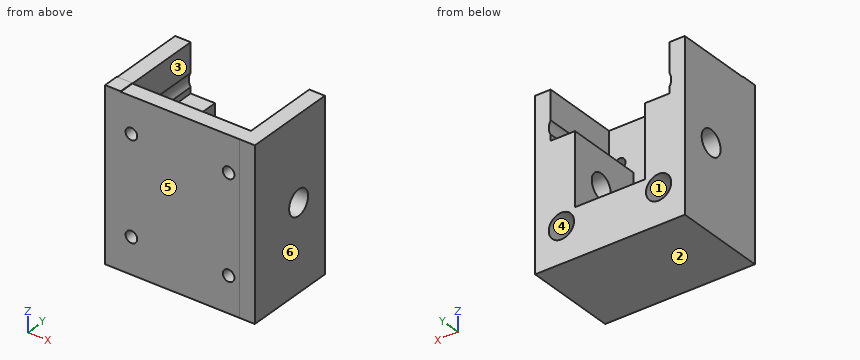
Autodesk Inventor part; units mm, degrees
ref_plane "Work Plane1" through (-15.25, 11.25, -51.1) normal (0, 1, 0) x (1, 0, 0)
ref_plane "Work Plane2" through (-15.25, 11.25, -7.7) normal (-1, 0, 0) x (0, 0, 1)
ref_plane "Work Plane3" through (15.25, 11.25, -51.1) normal (1, 0, 0) x (0, 0, -1)
ref_plane "Work Plane1" through (-15.25, 11.25, -51.1) normal (0, 1, 0) x (1, 0, 0)
sketch "Sketch1" plane through (-15.25, 11.25, -51.1) normal (0, 1, 0) x (1, 0, 0)
  line L0 (0, 0) -> (-1, 0)
  line L1 (30.5, 0) -> (30.5, -43.4)
  line L2 (0, 0) -> (30.5, 0)
  line L3 (30.5, 0) -> (30.5, -43.4)
  line L4 (30.5, -43.4) -> (0, -43.4)
  line L5 (0, -43.4) -> (0, 0)
  circle A0 centre (2.75, -9.2) radius 1.5
  circle A1 centre (2.75, -9.2) radius 1.5
  circle A2 centre (2.75, -34.2) radius 1.5
  circle A3 centre (2.75, -34.2) radius 1.5
  circle A4 centre (27.75, -34.2) radius 1.5
  circle A5 centre (27.75, -34.2) radius 1.5
  circle A6 centre (27.75, -9.2) radius 1.5
  circle A7 centre (27.75, -9.2) radius 1.5
  point P0 (15.25, -51.1)
extrude "Extrusion1" add sketch "Sketch1" along normal blind 4
ref_plane "Work Plane2" through (-15.25, 11.25, -7.7) normal (-1, 0, 0) x (0, 0, 1)
sketch "Sketch2" plane through (-15.25, 11.25, -7.7) normal (-1, 0, 0) x (0, 0, 1)
  line L0 (-43.4, 0) -> (-43.4, 4)
  line L1 (-43.4, 0) -> (0.1445, 0)
  line L2 (0.1445, 0) -> (0.1445, 4)
  line L3 (0.1445, 4) -> (-43.4, 4)
  line L4 (-43.4, 4) -> (-43.4, 0)
  point P0 (7.7, -11.25)
extrude "Extrusion2" add sketch "Sketch2" along normal blind 4
ref_plane "Work Plane3" through (15.25, 11.25, -51.1) normal (1, 0, 0) x (0, 0, -1)
sketch "Sketch3" plane through (15.25, 11.25, -51.1) normal (1, 0, 0) x (0, 0, -1)
  line L0 (0, 0) -> (0, 4)
  line L1 (0, 4) -> (-43.4, 4)
  line L2 (-43.4, 4) -> (-43.4, 0.0024)
  line L3 (-43.4, 0.0024) -> (0, 0.0024)
  line L4 (0, 0.0024) -> (0, 4)
  point P0 (-51.1, -11.25)
extrude "Extrusion3" add sketch "Sketch3" along normal blind 4
ref_plane "Work Plane6" through (-15.25, 15.25, -51.1) normal (0, 1, 0) x (1, 0, 0)
sketch "Sketch4" plane through (-15.25, 15.25, -51.1) normal (0, 1, 0) x (1, 0, 0)
  line L0 (-0.75, -43.4) -> (0.25, -43.4)
  line L1 (-0.0048, -43.4) -> (-4, -43.4)
  line L2 (-4, -43.4) -> (-4, 0)
  line L3 (-4, 0) -> (-0.0048, 0)
  line L4 (-0.0048, 0) -> (-0.0048, -43.4)
  point P0 (15.25, -51.1)
extrude "Extrusion4" add sketch "Sketch4" along normal blind 15
ref_plane "Work Plane5" through (-15.25, 15.25, -51.1) normal (0, 1, 0) x (1, 0, 0)
sketch "Sketch5" plane through (-15.25, 15.25, -51.1) normal (0, 1, 0) x (1, 0, 0)
  line L0 (30.5, 0) -> (34.5, 0)
  line L1 (30.5, -43.4) -> (30.5, 0)
  line L2 (34.5, 0) -> (30.5, 0)
  line L3 (30.5, 0) -> (30.5, -43.4)
  line L4 (30.5, -43.4) -> (34.5, -43.4)
  line L5 (34.5, -43.4) -> (34.5, 0)
  point P0 (15.25, -51.1)
extrude "Extrusion5" add sketch "Sketch5" along normal blind 15
ref_plane "Work Plane4" through (-15.25, 15.25, -51.1) normal (0, 1, 0) x (1, 0, 0)
sketch "Sketch6" plane through (-15.25, 15.25, -51.1) normal (0, 1, 0) x (1, 0, 0)
  circle A0 centre (2.75, -34.2) radius 2
  circle A1 centre (2.75, -34.2) radius 3.25
  circle A2 centre (27.75, -34.2) radius 1.5
  circle A3 centre (27.75, -34.2) radius 3.25
  circle A4 centre (27.75, -9.2) radius 1.5
  circle A5 centre (27.75, -9.2) radius 3.25
  circle A6 centre (2.75, -9.2) radius 1.5
  circle A7 centre (2.75, -9.2) radius 3.25
  line L0 (15.25, -21.7) -> (24.25, -21.7)
  line L1 (15.25, -21.7) -> (6.25, -21.7)
  line L2 (30.5, 0) -> (30.5, -43.4)
  line L3 (24.25, -21.7) -> (30.5, -21.7)
  line L4 (30.5, -21.7) -> (30.5, -12.45)
  line L5 (30.5, -12.45) -> (24.25, -12.45)
  line L6 (24.25, -12.45) -> (24.25, -21.7)
  line L7 (24.25, -21.7) -> (30.5, -21.7)
  line L8 (30.5, -21.7) -> (30.5, -30.95)
  line L9 (30.5, -30.95) -> (24.25, -30.95)
  line L10 (24.25, -30.95) -> (24.25, -21.7)
  line L11 (-0.0048, 0) -> (-0.0048, -43.4)
  line L12 (6.25, -21.7) -> (-0.0048, -21.7)
  line L13 (-0.0048, -21.7) -> (-0.0048, -30.95)
  line L14 (-0.0048, -30.95) -> (6.25, -30.95)
  line L15 (6.25, -30.95) -> (6.25, -21.7)
  line L16 (6.25, -21.7) -> (-0.0048, -21.7)
  line L17 (-0.0048, -21.7) -> (-0.0048, -12.45)
  line L18 (-0.0048, -12.45) -> (6.25, -12.45)
  line L19 (6.25, -12.45) -> (6.25, -21.7)
  point P0 (15.25, -51.1)
  dimension "d11" = 6.5
  dimension "d12" = 6.5
  dimension "d13" = 6.5
  dimension "d14" = 6.5
  dimension "d15" = 9
  dimension "d16" = 9
extrude "Extrusion6" add sketch "Sketch6" along normal blind 15 contours L6 L5 L2 L3 | L3 L2 L9 L10 | L14 L11 L12 L15 | L11 L18 L19 L12
ref_plane "Work Plane8" through (-15.25, 30.25, -51.1) normal (0, 1, 0) x (1, 0, 0)
sketch "Sketch7" plane through (-15.25, 30.25, -51.1) normal (0, 1, 0) x (1, 0, 0)
  line L0 (0, -43.4) -> (0, -43.5445)
  line L1 (-4, -43.4) -> (-0.0048, -43.4)
  line L2 (0, -43.4) -> (-4, -43.4)
  line L3 (-0.0048, 0) -> (-4, 0)
  line L4 (-4, -43.4) -> (-4, 0)
  line L5 (-4, 0) -> (-0.0048, 0)
  line L6 (-0.0048, -12.45) -> (-0.0048, 0)
  line L7 (-0.0048, 0) -> (-0.0048, -12.45)
  line L8 (6.25, -30.95) -> (6.25, -12.45)
  line L9 (-0.0048, -12.45) -> (6.25, -12.45)
  line L10 (6.25, -12.45) -> (6.25, -30.95)
  line L11 (-0.0048, -30.95) -> (-0.0048, -43.4)
  line L12 (6.25, -30.95) -> (-0.0048, -30.95)
  line L13 (-0.0048, -30.95) -> (-0.0048, -43.4)
  line L14 (24.25, -12.45) -> (24.25, -30.95)
  line L15 (24.25, -30.95) -> (24.25, -12.45)
  line L16 (30.5, -12.45) -> (24.25, -12.45)
  line L17 (24.25, -12.45) -> (30.5, -12.45)
  line L18 (30.5, -12.45) -> (30.5, 0)
  line L19 (30.5, 0) -> (34.4541, 0)
  line L20 (34.4541, 0) -> (34.4541, -43.4)
  line L21 (34.4541, -43.4) -> (30.5, -43.4)
  line L22 (30.5, -43.4) -> (30.5, -30.95)
  line L23 (30.5, -30.95) -> (24.25, -30.95)
  point P0 (15.25, -51.1)
extrude "Extrusion7" add sketch "Sketch7" along normal blind 5
ref_plane "Work Plane7" through (-15.25, 30.25, -51.1) normal (0, 1, 0) x (1, 0, 0)
sketch "Sketch8" plane through (-15.25, 30.25, -51.1) normal (0, 1, 0) x (1, 0, 0)
  line L0 (30.5, -43.4) -> (34.5, -43.4)
  line L1 (34.4541, 0) -> (34.4541, -43.4)
  line L2 (34.5, -43.4) -> (34.4541, -43.4)
  line L3 (34.4541, -43.4) -> (34.4541, 0)
  line L4 (34.4541, 0) -> (34.5, 0)
  line L5 (34.5, 0) -> (34.5, -43.4)
  point P0 (15.25, -51.1)
extrude "Extrusion8" add sketch "Sketch8" along normal blind 5
ref_plane "Work Plane9" through (-15.2548, 15.25, -38.65) normal (1, 0, 0) x (0, 0, -1)
sketch "Sketch9" plane through (-15.2548, 15.25, -38.65) normal (1, 0, 0) x (0, 0, -1)
  line L0 (0, 0) -> (0, 20)
  line L1 (12.45, 20) -> (0, 20)
  line L2 (0, 0) -> (12.45, 0)
  line L3 (12.45, 0) -> (12.45, 20)
  line L4 (12.45, 20) -> (0, 20)
  line L5 (0, 20) -> (0, 0)
  point P0 (-38.65, -15.25)
extrude "Extrusion9" add sketch "Sketch9" along normal up to surface (30.5048 mm away)
sketch "Sketch10" plane through (-15.25, 11.25, -51.1) normal (0, -1, 0) x (1, 0, 0)
  circle A0 centre (27.75, 9.2) radius 1.5
  circle A1 centre (27.75, 9.2) radius 1.5
  circle A2 centre (2.75, 9.2) radius 1.5
  circle A3 centre (2.75, 9.2) radius 1.5
  point P0 (15.25, 51.1)
extrude "Extrusion10" cut sketch "Sketch10" against normal through all
sketch "Sketch11" plane through (-15.25, 35.25, -51.1) normal (0, 1, 0) x (1, 0, 0)
  circle A0 centre (2.75, -9.2) radius 1.5
  circle A1 centre (2.75, -9.2) radius 3.25
  circle A2 centre (27.75, -9.2) radius 1.5
  circle A3 centre (27.75, -9.2) radius 3.25
  circle A4 centre (2.75, -34.2) radius 1.5
  circle A5 centre (2.75, -34.2) radius 3.25
  circle A6 centre (27.75, -34.2) radius 1.5
  circle A7 centre (27.75, -34.2) radius 3.25
  point P0 (15.25, -51.1)
  dimension "d27" = 6.5
  dimension "d28" = 6.5
  dimension "d29" = 6.5
  dimension "d30" = 6.5
extrude "Extrusion11" cut sketch "Sketch11" against normal up to surface (20 mm away) contours A0 | A1 | A2 | A3 | A4 | A5 | A6 | A7
sketch "Sketch12" plane through (9, 15.25, -20.15) normal (-1, 0, 0) x (0, 0, 1)
  line L0 (0, 20) -> (0, 0)
  line L1 (0, 20) -> (0, 11)
  line L2 (0, 11) -> (-9, 11)
  circle A0 centre (-9, 11) radius 3.25
  point P0 (20.15, -15.25)
  dimension "d33" = 9
  dimension "d34" = 9
  dimension "d35" = 6.5
extrude "Extrusion12" cut sketch "Sketch12" along normal mid plane 70
properties part number "linrail_mov_holder_ax"
Source: CAD feature listing. Evaluate the final solid. Frame: model axes, mm. Face numbers are marked on the shaded views. A direction names the side the tool comes from. Round coordinates to 2 decimals unless told otherwise and drop trailing zeros. Loops run counter-clockwise (first coordinate to the right, second up) from the corner with the lowest first, then second, coordinate; pieces in that order, holes last. Notation, with made-up numbers: M 27.5,-11.5 L 41.5,-11.5 A21 ccw 41.5,2.5 Z; hole C -8,19.25 d5. An arc over 180 degrees is marked long. Use a Markdown table: item, result. Add a question column.
1. Cut plane D-D, the plane y = 30.75. Output: boundary loops of the cut face in (x, z).
2. Cut plane A-A, the plane y = 26.25. Output: boundary loops of the cut face in (x, z).
3. Ray query, line 1 along X through (y, z) = (29.25, -41.9); line 2 along Z through (x, y) = (-12.5, 13.6); line 3 along X through (y, z) = (13.95, -41.9). Return the intervals inside material, ascending. Write a range as [from, to].
4. Cut plane C-C, the plane x = -12.5. Output: boundary loops of the cut face in (y, z), and give its area (3 significant figures).
5. Pull-direction query (X, two-part tool) for the marked faces 4, 5 and 6; classes: +X half, -X half, draft (parallel to the pull), parting line (faces both ways), or undercut.
6. Cut plane B-B, the plane z = -29.15. State how many separate pieces and enclosed holes the cut face has, and give its area (3 significant figures).
7. Set-up query: the marked faces 1, 2 and 3. Return all of +Z, -Z, +X, -X, +Y, -Y with unobstructed straight access to the full face (end or side cutting, diameter ignored); none if empty.
8. Contact query for flat-ended pins moving along their axis: pin 1 (7 mm diameter, centred on x = -12, z = -43, fed in from +Y); pin 2 (5 mm diameter, centred on x = -12, y = 23, fed in from +Z); pin 3 (1.2 mm diameter, centred on x = -16.5, y = 29.5, fed in from +Z); pin 4 (2.5 mm diameter, centred on x = 12.5, z = -41.9, fed in from +Y). Output: stop coordinate, or through.
Solution:
| question | item | result |
|---|---|---|
| 1 | outline | M -19.25,-51.1 L 19.25,-51.1 L 19.25,-7.7 L 15.25,-7.7 L 15.25,-15.17 A3.25 cw 15.25,-18.63 L 15.25,-20.15 L 9,-20.15 L 9,-38.65 L -9,-38.65 L -9,-20.15 L -15.25,-20.15 L -15.25,-18.62 A3.25 cw -15.25,-15.18 L -15.25,-7.7 L -19.25,-7.7 Z; hole C -12.5,-41.9 d6.5; hole C 12.5,-41.9 d6.5 |
| 2 | outline | M -19.25,-51.1 L 19.25,-51.1 L 19.25,-32.4 L 9,-32.4 L 9,-38.65 L -9,-38.65 L -9,-32.4 L -19.25,-32.4 Z; M -19.25,-25.9 L -9,-25.9 L -9,-20.15 L -15.25,-20.15 L -15.25,-18.62 A3.25 cw -15.25,-15.18 L -15.25,-7.7 L -19.25,-7.7 Z; M 9,-25.9 L 19.25,-25.9 L 19.25,-7.7 L 15.25,-7.7 L 15.25,-15.17 A3.25 cw 15.25,-18.63 L 15.25,-20.15 L 9,-20.15 Z; hole C -12.5,-41.9 d6.5; hole C 12.5,-41.9 d6.5 |
| 3 | line 1 | x = [-19.25, -15.75], [-9.25, 9.25], [15.75, 19.25] |
| 3 | line 2 | z = [-51.1, -43.4], [-40.4, -18.4], [-15.4, -7.7] |
| 3 | line 3 | x = [-19.25, -14], [-11, 11], [14, 19.25] |
| 4 | outline | M 11.25,-51.1 L 35.25,-51.1 L 35.25,-45.15 L 15.25,-45.15 L 15.25,-43.4 L 11.25,-43.4 Z; M 11.25,-40.4 L 15.25,-40.4 L 15.25,-38.65 L 35.25,-38.65 L 35.25,-20.15 L 15.25,-20.15 L 15.25,-18.4 L 11.25,-18.4 Z; M 11.25,-15.4 L 15.25,-15.4 L 15.25,-7.7 L 11.25,-7.7 Z; hole C 26.25,-29.15 d6.5 |
| 4 | area | 605 mm2 |
| 5 | face 4 | undercut |
| 5 | face 5 | draft |
| 5 | face 6 | +X half |
| 6 | separate pieces | 3 |
| 6 | enclosed holes | 0 |
| 6 | area | 431 mm2 |
| 7 | face 1 | +Y |
| 7 | face 2 | -Z, +X, -X, +Y, -Y |
| 7 | face 3 | +Z, +Y |
| 8 | pin 1 | stops at y = 35.25 |
| 8 | pin 2 | stops at z = -20.15 |
| 8 | pin 3 | stops at z = -7.7 |
| 8 | pin 4 | passes through |
